Verification items for the finished model (mm, model axes). Round coordinates to 2 decimals unless told otherwise and drop trailing zeros. Loops run counter-clockwise (first coordinate to the right, second up) from the corner with the lowest first, then second, coordinate; pieces in that order, holes last. Notation, with made-up numbers: M 81,-25.5 L 92,-25.5 A36 ccw 92,10.5 Z; hole C 2,73.5 d2. An arc over 180 degrees is marked long. One line per item, written item: value.
from build123d import *

# Parameters (mm, degrees)
F1_DEPTH = 1752.6
F3_DEPTH = 882.651
F6_DEPTH = 882.651
F7_DEPTH = 1525.507545


with BuildPart() as f1:
    # F0 (on Top) → F1 (new body)
    with BuildSketch(Plane.XY):
        with BuildLine():
            Line((879.29125, 0), (879.29125, 76.928016))
            ThreePointArc((879.29125, 76.928016), (0, 882.65), (-879.29125, 76.928016))
            Line((-879.29125, 76.928016), (-879.29125, 0))
            Line((-879.29125, 0), (879.29125, 0))
        make_face()
        with BuildLine():
            ThreePointArc((-872.965414, 76.374577), (0, 876.3), (872.965414, 76.374577))
            Line((872.965414, 76.374577), (872.965414, 21.737557))
            Line((872.965414, 21.737557), (-872.965414, 21.737557))
            Line((-872.965414, 21.737557), (-872.965414, 76.374577))
        make_face(mode=Mode.SUBTRACT)
    extrude(amount=F1_DEPTH)

    # F2 (on face) → F3 (cut, through all)
    with BuildSketch(Plane.XZ):
        Polygon((-914.4, 1821.486473), (-914.4, 1549.4), (914.4, 304.8), (994.86959, 1821.486473), align=None)
    extrude(amount=-F3_DEPTH, mode=Mode.SUBTRACT)

    # F4 (on face) → F6 (cut, through all)
    with BuildSketch(Plane.XZ):
        Polygon((857.237397, 220.805971), (-914.4, 1426.503644), (-914.4, 0), (914.4, 0), (914.4, 181.903644), align=None)
    extrude(amount=-F6_DEPTH, mode=Mode.SUBTRACT)

    # F5 (on Top) → F7 (cut, through all)
    with BuildSketch(Plane.XY):
        Polygon((-1011.60562, 79.864599), (-1011.60562, 0), (1011.60562, 0), (1018.673658, 79.864599), align=None)
    extrude(amount=F7_DEPTH, mode=Mode.SUBTRACT)


solid = f1.part
(1) Sectioned sample at D-D on x = 359.5. Enter the section's corners in (y, z), and give its area (3 significant figures).
Completed:
outline: M 799.16,559.54 L 806.12,559.54 L 806.12,682.44 L 799.16,682.44 Z
area: 855 mm^2
(2) Sectioned sample at B-B on y = 585. Enter the section's corners in (x, z), and give its area (3 significant figures).
Completed:
outline: M -660.94,1254.01 L -652.44,1248.22 L -652.44,1371.12 L -660.94,1376.91 Z; M 652.44,360.18 L 660.94,354.4 L 660.94,477.29 L 652.44,483.08 Z
area: 2,090 mm^2
(3) Sectioned sample at C-C on z = 816.5. Enter the section's corners in (x, y).
Completed:
outline: M -18.07,876.11 A876.3 cw 162.51,861.1 L 162.51,867.56 A882.65 ccw -18.07,882.47 Z
(4) Thickness scan on L1, parallel to Y at x = -295.5, z = 1034.5; L2, parallel to Z at x = -709, y = 519; L3, parallel to X at y = 382, z = 1455.5. Record the ranges inside material, lowest first. Write a range as from..to.
Completed:
L1: y = 824.97..831.72
L2: z = 1286.72..1409.61
L3: x = -795.71..-788.66
(5) Sectioned sample at A-A on y = 310.5. Enter the section's corners in (x, z), and give its area (3 significant figures).
Completed:
outline: M -826.23,1366.5 L -819.45,1361.88 L -819.45,1484.78 L -826.23,1489.4 Z; M 819.45,246.53 L 826.23,241.91 L 826.23,364.8 L 819.45,369.42 Z
area: 1,670 mm^2
